Autodesk Inventor part; units mm, degrees
ref_plane "YZ Plane" through (0, 0, 0) normal (1, 0, 0) x (0, 1, 0)
ref_plane "XZ Plane" through (0, 0, 0) normal (0, 1, 0) x (-1, 0, 0)
ref_plane "XY Plane" through (0, 0, 0) normal (0, 0, 1) x (1, 0, 0)
sketch "Sketch1" plane through (0, 0, 0) normal (0, 1, 0) x (-1, 0, 0)
  circle A0 centre (0, 0) radius 25
  dimension "d0" = 50
extrude "Extrusion1" add sketch "Sketch1" along normal blind 4.5
sketch "Sketch2" plane through (0, 4.5, 0) normal (0, 1, 0) x (1, 0, 0)
  line L0 (0, 0) -> (0, -22) construction
  circle A0 centre (0, -22) radius 1.6
  circle A1 centre (19.0526, -11) radius 1.6
  circle A2 centre (19.0526, 11) radius 1.6
  circle A3 centre (0, 22) radius 1.6
  circle A4 centre (-19.0526, 11) radius 1.6
  circle A5 centre (-19.0526, -11) radius 1.6
  dimension "d3" = 22
  dimension "d4" = 3.2
  dimension "d7" = 360
extrude "Extrusion2" cut sketch "Sketch2" against normal up to surface (4.5 mm away)
sketch "Sketch3" plane through (0, 4.5, 0) normal (0, 1, 0) x (1, 0, 0)
  line L0 (0, 0) -> (0, -11)
  line L1 (0, 0) -> (11, 0) construction
  circle A0 centre (0, -11) radius 1.35
  circle A1 centre (7.7782, -7.7782) radius 1.35
  circle A2 centre (11, 0) radius 1.35
  circle A3 centre (7.7782, 7.7782) radius 1.35
  circle A4 centre (0, 11) radius 1.35
  circle A5 centre (-7.7782, 7.7782) radius 1.35
  circle A6 centre (-11, 0) radius 1.35
  circle A7 centre (-7.7782, -7.7782) radius 1.35
  dimension "d11" = 11
  dimension "d12" = 90
  dimension "d13" = 2.7
  dimension "d16" = 360
extrude "Extrusion3" cut sketch "Sketch3" against normal up to surface (4.5 mm away)
sketch "Sketch4" plane through (0, 0, 0) normal (0, -1, 0) x (1, 0, 0)
  circle A0 centre (-11, 0) radius 1.35 construction
  circle A1 centre (-7.7782, 7.7782) radius 1.35 construction
  circle A2 centre (-7.7782, -7.7782) radius 1.35 construction
  circle A3 centre (7.7782, -7.7782) radius 1.35 construction
  circle A4 centre (7.7782, 7.7782) radius 1.35 construction
  circle A5 centre (0, 11) radius 1.35 construction
  circle A6 centre (11, 0) radius 1.35 construction
  circle A7 centre (0, -11) radius 1.35 construction
  circle A8 centre (-19.0526, -11) radius 1.6 construction
  circle A9 centre (-19.0526, 11) radius 1.6 construction
  circle A10 centre (0, -22) radius 1.6 construction
  circle A11 centre (19.0526, 11) radius 1.6 construction
  circle A12 centre (0, 22) radius 1.6 construction
  circle A13 centre (19.0526, -11) radius 1.6 construction
  circle A14 centre (0, 0) radius 25 construction
  line L0 (0, 0) -> (0, -8.5) construction
  line L1 (1.4434, -8.5) -> (2.8868, -11)
  line L2 (2.8868, -11) -> (1.4434, -13.5)
  line L3 (1.4434, -13.5) -> (-1.4434, -13.5)
  line L4 (-1.4434, -13.5) -> (-2.8868, -11)
  line L5 (-2.8868, -11) -> (-1.4434, -8.5)
  line L6 (-1.4434, -8.5) -> (1.4434, -8.5)
  line L7 (5.7369, -9.8194) -> (4.9898, -7.031)
  line L8 (8.5253, -10.5666) -> (5.7369, -9.8194)
  line L9 (10.5666, -8.5253) -> (8.5253, -10.5666)
  line L10 (9.8194, -5.7369) -> (10.5666, -8.5253)
  line L11 (7.031, -4.9898) -> (9.8194, -5.7369)
  line L12 (4.9898, -7.031) -> (7.031, -4.9898)
  line L13 (11, -2.8868) -> (8.5, -1.4434)
  line L14 (13.5, -1.4434) -> (11, -2.8868)
  line L15 (13.5, 1.4434) -> (13.5, -1.4434)
  line L16 (11, 2.8868) -> (13.5, 1.4434)
  line L17 (8.5, 1.4434) -> (11, 2.8868)
  line L18 (8.5, -1.4434) -> (8.5, 1.4434)
  line L19 (9.8194, 5.7369) -> (7.031, 4.9898)
  line L20 (10.5666, 8.5253) -> (9.8194, 5.7369)
  line L21 (8.5253, 10.5666) -> (10.5666, 8.5253)
  line L22 (5.7369, 9.8194) -> (8.5253, 10.5666)
  line L23 (4.9898, 7.031) -> (5.7369, 9.8194)
  line L24 (7.031, 4.9898) -> (4.9898, 7.031)
  line L25 (2.8868, 11) -> (1.4434, 8.5)
  line L26 (1.4434, 13.5) -> (2.8868, 11)
  line L27 (-1.4434, 13.5) -> (1.4434, 13.5)
  line L28 (-2.8868, 11) -> (-1.4434, 13.5)
  line L29 (-1.4434, 8.5) -> (-2.8868, 11)
  line L30 (1.4434, 8.5) -> (-1.4434, 8.5)
  line L31 (-5.7369, 9.8194) -> (-4.9898, 7.031)
  line L32 (-8.5253, 10.5666) -> (-5.7369, 9.8194)
  line L33 (-10.5666, 8.5253) -> (-8.5253, 10.5666)
  line L34 (-9.8194, 5.7369) -> (-10.5666, 8.5253)
  line L35 (-7.031, 4.9898) -> (-9.8194, 5.7369)
  line L36 (-4.9898, 7.031) -> (-7.031, 4.9898)
  line L37 (-11, 2.8868) -> (-8.5, 1.4434)
  line L38 (-13.5, 1.4434) -> (-11, 2.8868)
  line L39 (-13.5, -1.4434) -> (-13.5, 1.4434)
  line L40 (-11, -2.8868) -> (-13.5, -1.4434)
  line L41 (-8.5, -1.4434) -> (-11, -2.8868)
  line L42 (-8.5, 1.4434) -> (-8.5, -1.4434)
  line L43 (-9.8194, -5.7369) -> (-7.031, -4.9898)
  line L44 (-10.5666, -8.5253) -> (-9.8194, -5.7369)
  line L45 (-8.5253, -10.5666) -> (-10.5666, -8.5253)
  line L46 (-5.7369, -9.8194) -> (-8.5253, -10.5666)
  line L47 (-4.9898, -7.031) -> (-5.7369, -9.8194)
  line L48 (-7.031, -4.9898) -> (-4.9898, -7.031)
  point P0 (6.0104, -6.0104)
  point P1 (8.5, 0)
  point P2 (6.0104, 6.0104)
  point P3 (0, 8.5)
  point P4 (-6.0104, 6.0104)
  point P5 (-8.5, 0)
  point P6 (-6.0104, -6.0104)
  dimension "d20" = 8.5
  dimension "d23" = 360
extrude "Extrusion4" cut sketch "Sketch4" against normal blind 2
sketch "Sketch5" plane through (0, 4.5, 0) normal (0, 1, 0) x (1, 0, 0)
  circle A0 centre (-11, 0) radius 1.35 construction
  circle A1 centre (-7.7782, -7.7782) radius 1.35 construction
  circle A2 centre (-7.7782, 7.7782) radius 1.35 construction
  circle A3 centre (7.7782, 7.7782) radius 1.35 construction
  circle A4 centre (7.7782, -7.7782) radius 1.35 construction
  circle A5 centre (0, -11) radius 1.35 construction
  circle A6 centre (11, 0) radius 1.35 construction
  circle A7 centre (0, 11) radius 1.35 construction
  circle A8 centre (-19.0526, 11) radius 1.6 construction
  circle A9 centre (-19.0526, -11) radius 1.6 construction
  circle A10 centre (0, 22) radius 1.6 construction
  circle A11 centre (19.0526, -11) radius 1.6 construction
  circle A12 centre (0, -22) radius 1.6 construction
  circle A13 centre (19.0526, 11) radius 1.6 construction
  circle A14 centre (0, 0) radius 25 construction
  circle A15 centre (0, -22) radius 2.35
  circle A16 centre (19.0526, -11) radius 2.35
  circle A17 centre (19.0526, 11) radius 2.35
  circle A18 centre (0, 22) radius 2.35
  circle A19 centre (-19.0526, 11) radius 2.35
  circle A20 centre (-19.0526, -11) radius 2.35
  dimension "d27" = 4.7
  dimension "d30" = 360
extrude "Extrusion5" cut sketch "Sketch5" against normal blind 2.6
sketch "Sketch6" plane through (0, 4.5, 0) normal (0, 1, 0) x (1, 0, 0)
  circle A0 centre (0, 0) radius 2.8
  dimension "d34" = 5.6
extrude "Extrusion6" cut sketch "Sketch6" against normal up to surface (4.5 mm away)
sketch "Sketch7" plane through (0, 4.5, 0) normal (0, 1, 0) x (1, 0, 0)
  circle A0 centre (-19.0526, 11) radius 2.35 construction
  circle A1 centre (19.0526, 11) radius 2.35 construction
  circle A2 centre (0, -22) radius 2.35 construction
  circle A3 centre (19.0526, -11) radius 2.35 construction
  circle A4 centre (0, 22) radius 2.35 construction
  circle A5 centre (-19.0526, -11) radius 2.35 construction
  circle A6 centre (-11, 0) radius 1.35 construction
  circle A7 centre (-7.7782, -7.7782) radius 1.35 construction
  circle A8 centre (-7.7782, 7.7782) radius 1.35 construction
  circle A9 centre (7.7782, 7.7782) radius 1.35 construction
  circle A10 centre (7.7782, -7.7782) radius 1.35 construction
  circle A11 centre (0, -11) radius 1.35 construction
  circle A12 centre (11, 0) radius 1.35 construction
  circle A13 centre (0, 11) radius 1.35 construction
  circle A14 centre (0, 0) radius 25 construction
  line L0 (0, -22) -> (0, -18) construction
  line L1 (0, -18) -> (2.1213, -15.8787)
  line L2 (0, -18) -> (3, -18) construction
  line L3 (2.1213, -15.8787) -> (0.6213, -15.8787)
  line L4 (0.6213, -15.8787) -> (0.6213, -12.8787)
  line L5 (0.6213, -12.8787) -> (0.2071, -12.8787)
  line L6 (0, -18) -> (-2.1213, -15.8787)
  line L7 (-2.1213, -15.8787) -> (-0.6213, -15.8787)
  line L8 (-0.6213, -15.8787) -> (-0.6213, -12.8787)
  line L9 (-0.6213, -12.8787) -> (0.2071, -12.8787)
  dimension "d37" = 4
  dimension "d38" = 3
  dimension "d39" = 45
  dimension "d40" = 1.5
  dimension "d41" = 45
  dimension "d42" = 3
extrude "Extrusion7" cut sketch "Sketch7" against normal blind 0.4
properties part number "sea_connector"
Verification items for the finished model (mm, model axes). A direction names the side the tool comes from. Round coordinates to 2 decimals unless told otherwise and drop trailing zeros. Order: outer loops, then holes, each group sorted by start corner. A loop starts at its lowest first (then second) coordinate and runs counter-clockwise, first axis right, second up.
1. Section check B-B on z = -22. Record the cut outline in (x, y).
Final values:
outline: (-11.87, 0) - (-1.6, 0) - (-1.6, 1.9) - (-2.35, 1.9) - (-2.35, 4.5) - (-11.87, 4.5) - close; (1.6, 0) - (11.87, 0) - (11.87, 4.5) - (2.35, 4.5) - (2.35, 1.9) - (1.6, 1.9) - close
2. Release check for a two-part mould opening along Z. For faces 4 (the flat face through (-1, 4.3, 17)), 5 (the flat face through (0, 1, 13.5)), 6 (the flat face through (0, 0, -5)) record: +Z half, -Z half, draft (parallel to the pull), parting line (faces both ways), or undercut.
Final values:
face 4: undercut
face 5: undercut
face 6: draft
3. Section check C-C on y = 1.2. State how many separate pieces and enclosed holes the cut face has, then the cut area to 3 significant figures.
Final values:
separate pieces: 1
enclosed holes: 15
area: 1,720 mm2
4. Thickness scan on L1, parallel to Z at x = 0, y = 3.95; L2, parallel to X at y = 1, z = 6; L3, parallel to X at y = 0.65, z = 7.5. Record the ranges inside material, lowest first.
Final values:
L1: z = -25 to -24.35, -19.65 to -12.35, -9.65 to -2.8, 2.8 to 9.65, 12.35 to 19.65, 24.35 to 25
L2: x = -24.27 to -9.89, -6.02 to 6.02, 9.89 to 24.27
L3: x = -23.85 to -10.29, -5.12 to 5.12, 10.29 to 23.85
5. Go/stop test with flat-tipped pins: P1, Ø3.5, axis at x = -7.78, z = 7.78, coming from the -Y side; P2, Ø4, axis at x = 0, z = -22, coming from the -Y side; P3, Ø2, axis at x = -10.5, y = 3, coming from the +Z side; P4, Ø2.5, axis at x = -7.78, z = -7.78, coming from the -Y side. Record where each tip stops, or that it passes through.
Final values:
P1: stops at y = 2
P2: stops at y = 0
P3: stops at z = 23.12
P4: passes through
6. Access from +Z, -Z, +X, -X, +Y, -Y to the whole of each face (thin tool, end or side, straight path). Record for faces 1 (the flat face through (0, 1, 8.5)), 2 (the cylindrical face through (17.87, 0.96, -12.08)), 3 (the flat face through (0, 1.9, 24)).
Final values:
face 1: -Y
face 2: +Y, -Y
face 3: +Y
7. Section check A-A on z = 0. Record the cut outline in (x, y), then the cut area to 3 significant figures.
Final values:
outline: (-25, 0) - (-13.5, 0) - (-13.5, 2) - (-12.35, 2) - (-12.35, 4.5) - (-25, 4.5) - close; (-9.65, 2) - (-8.5, 2) - (-8.5, 0) - (-2.8, 0) - (-2.8, 4.5) - (-9.65, 4.5) - close; (2.8, 0) - (8.5, 0) - (8.5, 2) - (9.65, 2) - (9.65, 4.5) - (2.8, 4.5) - close; (12.35, 2) - (13.5, 2) - (13.5, 0) - (25, 0) - (25, 4.5) - (12.35, 4.5) - close
area: 166 mm2
